Work out the finished part from the listing and answer in its coordinate system (mm). A direction names the side the tool comes from. Give positions to 0.01 mm unless a question says otherwise; leave off trailing zeros. Order: outer loops, then holes, each group sorted by start corner. A loop starts at its lowest first (then second) coordinate and runs counter-clockwise, first axis right, second up. Notation, with made-up numbers: (66.25, 25) - (100.25, 25) arc R24 cw to (100.25, 63) - close; hole circle Ø1 at (51, -35.75). An arc over 180 degrees is marked (long way). Return JSON: item names as keys, results as strings. Group by question number.
from build123d import *

# Parameters (mm, degrees)
SALIENTE_EXTRUIR3_DEPTH      = 110
SALIENTE_EXTRUIR3_DEPTH_BACK = 10
CORTAR_EXTRUIR3_START        = -3
CORTAR_EXTRUIR3_OUTLINE_R    = 3
CORTAR_EXTRUIR3_DEPTH        = 22.583018394


# Read off the part's stored shape, not the designer's step: Cortar-Extruir3
with BuildPart() as part:
    # Croquis9 → Saliente-Extruir3 (new, two sides: drawn at the far end of the back side and taken through both)
    with BuildSketch(Plane(origin=(0, 0, 0), x_dir=(0, 0, -1), z_dir=(1, 0, 0)).offset(-SALIENTE_EXTRUIR3_DEPTH_BACK)):
        with BuildLine():
            Line((5.538630524, -12.462), (5.538630524, 50.038))
            Line((5.538630524, 50.038), (-14.04438787, 87.324884341))
            Line((-14.04438787, 87.324884341), (-14.04438787, 93.670477998))
            Line((-14.04438787, 93.670477998), (-14.04438787, 105.09803176))
            ThreePointArc((-14.04438787, 105.09803176), (-12.54438787, 106.59803176), (-11.04438787, 105.09803176))
            Line((-11.04438787, 105.09803176), (-11.04438787, 93.670477998))
            Line((-11.04438787, 93.670477998), (-11.04438787, 88.064764588))
            Line((-11.04438787, 88.064764588), (8.538630524, 50.777880247))
            Line((8.538630524, 50.777880247), (8.538630524, -12.462))
            ThreePointArc((8.538630524, -12.462), (7.038630524, -13.962), (5.538630524, -12.462))
        make_face()
    extrude(amount=SALIENTE_EXTRUIR3_DEPTH + SALIENTE_EXTRUIR3_DEPTH_BACK)

    # Cortar-Extruir3 outline → Cortar-Extruir3 (cut)
    with BuildSketch(Plane.XY.offset(-5.538630524).offset(CORTAR_EXTRUIR3_START)):
        Polygon((91.833498399, 4.799000122), (91.833498399, 19.839000383), (85.846003394, 19.839000122), (85.846004052, 4.799000122), align=None)
        with Locations((20.066122073, 6.603918538)):
            Circle(CORTAR_EXTRUIR3_OUTLINE_R)
        with Locations((29.845121402, 6.476918682)):
            Circle(CORTAR_EXTRUIR3_OUTLINE_R)
        Polygon((59.620998024, 34.067003823), (32.620998024, 34.067001462), (32.620998024, 15.367003823), (59.620998024, 15.367003823), align=None)
        with BuildLine():
            Line((92.16369837, 28.270001136), (92.163697895, 33.705601107))
            ThreePointArc((92.163697895, 33.705601107), (92.066984544, 33.939087777), (91.833497866, 34.035801107))
            Line((91.833497866, 34.035801107), (86.397897866, 34.035800632))
            ThreePointArc((86.397897866, 34.035800632), (86.164411215, 33.939087271), (86.067697895, 33.705600603))
            Line((86.067697895, 33.705600603), (86.06769837, 28.270000603))
            ThreePointArc((86.06769837, 28.270000603), (86.164411732, 28.036513952), (86.397898399, 27.939800632))
            Line((86.397898399, 27.939800632), (91.833498399, 27.939801107))
            ThreePointArc((91.833498399, 27.939801107), (92.066985049, 28.036514469), (92.16369837, 28.270001136))
        make_face()
        with Locations((38.35412218, 6.603918538)):
            Circle(CORTAR_EXTRUIR3_OUTLINE_R)
        with Locations((53.339878017, 92.075080872)):
            Circle(CORTAR_EXTRUIR3_OUTLINE_R)
    extrude(amount=CORTAR_EXTRUIR3_DEPTH, mode=Mode.SUBTRACT)


solid = part.part
1. A tool of negligible diameter and unlimited length cuts with its end or side. For faces 4 (the flat face through (49, 96, 14.044)), 5 (the flat face through (46, 15.367, -7)), 6 (the flat face through (49, 11, -5.539)), from which of +Z, -Z, +X, -X, +Y, -Y can it reach the whole face along a straight path? Write none if from no direction.
2. The part is cut by section B-B (x = 13). Give the vertices of the cut face in (y, z).
3. The part is cut by section A-A (y = 22). Give the vertices of the cut face in (x, z), and give its area (3 significant figures).
4. The part is cut by section C-C (y = 97.5). Give the vertices of the cut face in (x, z).
5. Consider probe 1 along X at (y, z) = (28.5, -6); probe 2 along Z at (x, y) = (62, 33); probe 3 along Z at (x, y) = (0, 91.5). Determine where each line is inside the solid, lowest interval first. Write a range as from..to.
6. The part is cut by section D-D (z = 0.5). Give the vertices of the cut face in (x, y).
7. Each of these flat-tipped pins is pushed along its axis until it touches: pin 1 (8.5 mm diameter, centred on x = 24, y = 95.5, fed in from -Z); pin 2 (1 mm diameter, centred on x = 63, y = 74, fed in from -Z) (3 decimals); pin 3 (9.5 mm diameter, centred on x = 38.35, y = 6.6, fed in from +Z). Where does it stop, or does it pass through?
8. Determine the mould class of faces 1 (the flat face through (85.846, 12, -7)), 2 (the flat face through (110, 47, -6)), 3 (the flat face through (49.2, 69.7, 1.4)) for opening direction X: released by +X, released by -X, zero draft, split by the parting line, or undercut.
Answers:
{
 "1": {"face 4": "+Z, +X, -X, +Y, -Y", "face 5": "+Z, -Z", "face 6": "+Z, +X, -X, -Y"},
 "2": {"outline": "(-12.46, -8.54) - (50.78, -8.54) - (88.06, 11.04) - (105.1, 11.04) arc R1.5 ccw to (105.1, 14.04) - (87.32, 14.04) - (50.04, -5.54) - (-12.46, -5.54) arc R1.5 ccw to start"},
 "3": {"outline": "(-10, -8.54) - (32.62, -8.54) - (32.62, -5.54) - (-10, -5.54) - close; (59.62, -8.54) - (110, -8.54) - (110, -5.54) - (59.62, -5.54) - close", "area": "279 mm^2"},
 "4": {"outline": "(-10, 11.04) - (110, 11.04) - (110, 14.04) - (-10, 14.04) - close"},
 "5": {"probe 1": "x = -10..32.62, 59.62..86.07, 92.16..110", "probe 2": "z = -8.54..-5.54", "probe 3": "z = 11.04..14.04"},
 "6": {"outline": "(-10, 61.54) - (110, 61.54) - (110, 67.99) - (-10, 67.99) - close"},
 "7": {"pin 1": "stops at z = 11.04", "pin 2": "stops at z = 3.395", "pin 3": "stops at z = -5.54"},
 "8": {"face 1": "undercut", "face 2": "released by +X", "face 3": "zero draft"}
}
